```python
from build123d import *

# Parameters (mm, degrees)
BOSS_EXTRUDE1_DEPTH = 70
SKETCH2_W           = 3
SKETCH2_H           = 70
BOSS_EXTRUDE2_DEPTH = 20
LPATTERN2_COUNT     = 2
LPATTERN2_PITCH     = 73
SKETCH3_W           = 70
SKETCH3_H           = 3
BOSS_EXTRUDE3_DEPTH = 20
LPATTERN3_COUNT     = 2
LPATTERN3_PITCH     = 70
SKETCH6_W           = 3
SKETCH6_H           = 70
BOSS_EXTRUDE4_DEPTH = 20
LPATTERN4_COUNT     = 2
LPATTERN4_PITCH     = 70
SKETCH8_W           = 70
SKETCH8_H           = 3
BOSS_EXTRUDE5_DEPTH = 20
LPATTERN5_COUNT     = 3
LPATTERN5_PITCH     = 70


with BuildPart() as part:
    # Sketch1 → Boss-Extrude1 (new body)
    with BuildSketch(Plane.XY):
        with BuildLine():
            Line((150, -5), (0, -5))
            ThreePointArc((0, -5), (-5, 0), (0, 5))
            Line((0, 5), (147.636546096, 5))
            Line((147.636546096, 5), (261.136368727, 143.173697117))
            ThreePointArc((261.136368727, 143.173697117), (268.173697117, 143.863631273), (268.863631273, 136.826302883))
            Line((268.863631273, 136.826302883), (153.863631273, -3.173697117))
            ThreePointArc((153.863631273, -3.173697117), (152.136763255, -4.520425068), (150, -5))
        make_face()
    extrude(amount=BOSS_EXTRUDE1_DEPTH)

    # Sketch2 → Boss-Extrude2 (add)
    with BuildSketch(Plane(origin=(0, 5, 0), x_dir=(1, 0, 0), z_dir=(0, 1, 0))):
        with Locations((10.170720814, -35)):
            Rectangle(SKETCH2_W, SKETCH2_H)
    boss_extrude2 = extrude(amount=BOSS_EXTRUDE2_DEPTH)

    # LPattern2: Boss-Extrude2 ×2
    with Locations(*[(i * LPATTERN2_PITCH, 0, 0) for i in range(1, LPATTERN2_COUNT)]):
        add(boss_extrude2)

    # Sketch3 → Boss-Extrude3 (add)
    with BuildSketch(Plane(origin=(85.702248392, -70.398275465, 0), x_dir=(0, 0, 1), z_dir=(-0.7727262545252344, 0.6347394233600138, 0))):
        with Locations((35, 154.104367408)):
            Rectangle(SKETCH3_W, SKETCH3_H)
    boss_extrude3 = extrude(amount=BOSS_EXTRUDE3_DEPTH)

    # LPattern3: Boss-Extrude3 ×2
    with Locations(*[Vector(0.6347394233600138, 0.7727262545252344, 0) * (i * LPATTERN3_PITCH) for i in range(1, LPATTERN3_COUNT)]):
        add(boss_extrude3)

    # Sketch6 → Boss-Extrude4 (add)
    with BuildSketch(Plane.XZ.offset(5)):
        with Locations((47.13, 35)):
            Rectangle(SKETCH6_W, SKETCH6_H)
    boss_extrude4 = extrude(amount=BOSS_EXTRUDE4_DEPTH)

    # LPattern4: Boss-Extrude4 ×2
    with Locations(*[(i * LPATTERN4_PITCH, 0, 0) for i in range(1, LPATTERN4_COUNT)]):
        add(boss_extrude4)

    # Sketch8 → Boss-Extrude5 (add)
    with BuildSketch(Plane(origin=(93.429510938, -76.745669699, 0), x_dir=(0, 0, -1), z_dir=(0.7727262545252342, -0.6347394233600141, 0))):
        with Locations((-35, 105.900913504)):
            Rectangle(SKETCH8_W, SKETCH8_H)
    boss_extrude5 = extrude(amount=BOSS_EXTRUDE5_DEPTH)

    # LPattern5: Boss-Extrude5 ×3
    with Locations(*[Vector(0.6347394233600141, 0.7727262545252341, 0) * (i * LPATTERN5_PITCH) for i in range(1, LPATTERN5_COUNT)]):
        add(boss_extrude5)


solid = part.part
```
The listing builds one solid part. Answer for the finished solid, in the listing's coordinates (mm). A direction names the side the tool comes from. Round coordinates to 2 decimals unless told otherwise and drop trailing zeros. Write each loop counter-clockwise with the first axis right and the second up, starting at its lowest first coordinate (ties: lowest second). Pieces come first, ordered by that corner, then holes. Notation, with made-up numbers: (27.5, 2) -> (47.5, 2) arc R26 ccw to (47.5, 32) -> close; hole circle Ø1 at (62.25, -30.5). An arc over 180 degrees is marked (long way). Use CSV: the item, a comma, the result in double quotes. Start each with the question number.
(1) Section A-A on y = 20 is taken. Give the vertices of the cut face in (x, z), then the cut area to 3 significant figures.
(2) Section C-C on y = 140 is taken. Give the vertices of the cut face in (x, z), then the cut area to 3 significant figures.
(3) Section D-D on y = 86.5 is taken. Give the vertices of the cut face in (x, z).
(4) Consider L1, parallel to X at y = -11, z = 18.5; L2, parallel to Y at x = 217, z = 58; L3, parallel to Y at x = 41, z = 58.5. Determine where each line is inside the solid, lowest interval first. Write a range as from..to.
(5) Each of these flat-tipped pins is pushed along its axis until it touches: pin 1 (7 mm diameter, centred on x = 2.5, z = 24, fed in from +Y); pin 2 (16 mm diameter, centred on y = -18.5, z = 18.5, fed in from -X); pin 3 (16 mm diameter, centred on y = 10.5, z = 52.5, fed in from -X). Where does it stop, or does it pass through?
(6) Which of the six approach directions +Z, -Z, +X, -X, +Y, -Y give full straight-line access (tool end or side, diameter ignored) to faces 1 (the face through (45.63, -15, 35)), 2 (the face through (8.671, 15, 35)), 3 (the face through (81.671, 15, 35))?
(7) The mould has two halves that part along Y. Classify faces 4 (the face through (46, 5, 35)), 5 (the face through (169.22, -0.01, 35.49)), 6 (the face through (83, -5, 35)): released by +Y, released by -Y, zero draft, split by the parting line, or undercut.
(8) Section B-B on y = 0 is taken. Give the vertices of the cut face in (x, z), then the cut area to 3 significant figures.
A:
1,outline,"(8.67, 0) -> (11.67, 0) -> (11.67, 70) -> (8.67, 70) -> close; (81.67, 0) -> (84.67, 0) -> (84.67, 70) -> (81.67, 70) -> close; (159.96, 0) -> (172.9, 0) -> (172.9, 70) -> (159.96, 70) -> close"
1,area,"1,330 mm²"
2,outline,"(258.53, 0) -> (270, 0) -> (270, 70) -> (258.53, 70) -> close"
2,area,"803 mm²"
3,outline,"(214.58, 0) -> (227.52, 0) -> (227.52, 70) -> (214.58, 70) -> close"
4,L1,"x = 45.63..48.63, 115.63..118.63"
4,L2,"y = 47.45..51.33, 73.69..89.44, 109.83..113.71"
4,L3,"y = -5..5"
5,pin 1,"stops at y = 5"
5,pin 2,"stops at x = 45.63"
5,pin 3,"stops at x = -4.33"
6,face 1,"+Z, -Z, -X, -Y"
6,face 2,"+Z, -Z, -X, +Y"
6,face 3,"+Z, -Z, +Y"
7,face 4,"released by +Y"
7,face 5,"undercut"
7,face 6,"released by -Y"
8,outline,"(-5, 0) -> (156.47, 0) -> (156.47, 70) -> (-5, 70) -> close; (164.48, 0) -> (169.2, 0) -> (169.2, 70) -> (164.48, 70) -> close"
8,area,"11,600 mm²"
